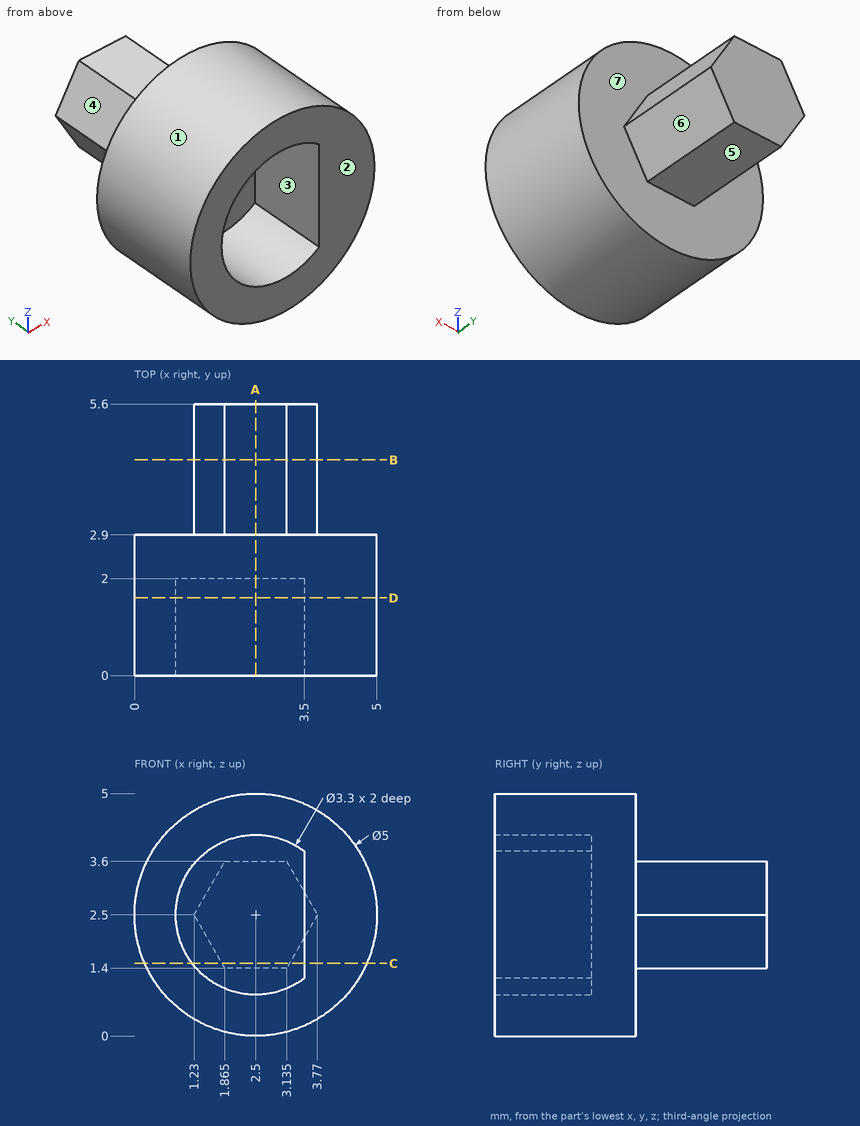
Geometry check sheet. Reference: drawing and pictorial views, mm from the part's lowest x, y, z. A direction names the side the tool comes from. Give positions to 0.01 mm unless a question says otherwise; leave off trailing zeros. Order: outer loops, then holes, each group sorted by start corner. A loop starts at its lowest first (then second) coordinate and runs counter-clockwise, first axis right, second up. Notation, with made-up numbers: (-21.5, -25.75) - (23.5, -25.75) arc R21 cw to (23.5, 8.25) - close; hole circle Ø2 at (34.5, 9). An arc over 180 degrees is marked (long way). Use one line per item in the form item = value.
1) Sectioned sample at D-D (y = 1.6). Record the boundary of the cut face in (x, z).
Working result:
outline = circle Ø5 at (2.5, 2.5); hole (3.5, 1.19) - (3.5, 3.81) arc R1.65 ccw (long way) to start
2) Material ranges on probe 1 along X at (y, z) = (1.5, 2.5); probe 2 along Z at (x, y) = (2.45, 3.2); probe 3 along Y at (x, z) = (2.3, 0.3), recorded low to high. Write a range as from..to.
Working result:
probe_1 = 0..0.85, 3.5..5
probe_2 = 1.4..3.6
probe_3 = 0..2.9
3) Draft check along Z on the marked faces 1, 2 and 3. Enter one of: released by +Z, released by -Z, zero draft, split by the parting line, or undercut.
Working result:
face_1 = split by the parting line
face_2 = zero draft
face_3 = undercut
4) Sectioned sample at C-C (z = 1.5). Record the boundary of the cut face in (x, y), and give its area (3 significant figures).
Working result:
outline = (0.21, 0) - (1.19, 0) - (1.19, 2) - (3.5, 2) - (3.5, 0) - (4.79, 0) - (4.79, 2.9) - (3.19, 2.9) - (3.19, 5.6) - (1.81, 5.6) - (1.81, 2.9) - (0.21, 2.9) - close
area = 12.4 mm^2
5) Depth check by flat-ended pin: pin 1 Ø1.5 at (x, z) = (1.5, 3.5) entering from +Y; pin 2 Ø1 at (x, y) = (2.5, 4) entering from -Z; pin 3 Ø3 at (y, z) = (0.5, 0.5) entering from -X; pin 4 Ø0.6 at (x, y) = (2.5, 4.5) entering from +Z. Enter the tip coordinate at first touch or a pass-through.
Working result:
pin_1 = 5.6
pin_2 = 1.4
pin_3 = 0.05
pin_4 = 3.6
6) Sectioned sample at A-A (x = 2.5). Record the boundary of the cut face in (y, z).
Working result:
outline = (0, 0) - (2.9, 0) - (2.9, 1.4) - (5.6, 1.4) - (5.6, 3.6) - (2.9, 3.6) - (2.9, 5) - (0, 5) - (0, 4.15) - (2, 4.15) - (2, 0.85) - (0, 0.85) - close
7) Access from +Z, -Z, +X, -X, +Y, -Y to the whole of each face (thin tool, end or side, straight path). Record for the marked faces 4, 5, 6 and 7.
Working result:
face_4 = +Z, -X, +Y
face_5 = -Z, +X, -X, +Y
face_6 = -Z, +X, +Y
face_7 = +Y
8) Sectioned sample at B-B (y = 4.45). Record the boundary of the cut face in (x, z) (1 decimal), and give its area (3 significant figures).
Working result:
outline = (1.2, 2.5) - (1.9, 1.4) - (3.1, 1.4) - (3.8, 2.5) - (3.1, 3.6) - (1.9, 3.6) - close
area = 4.19 mm^2
